```python
from build123d import *

# Parameters (mm, degrees)
BOSS_EXTRUDE1_DEPTH      = 2.5
CHAMFER1_SIZE            = 2.65
CHAMFER1_SIZE_2          = 0.5
FILLET1_R                = 0.254
REVOLVE1_ANGLE           = 180
REVOLVE1_OTHER_WAY_ANGLE = 180
SKETCH3_W                = 0.4
SKETCH3_H                = 0.76
BOSS_EXTRUDE2_DEPTH      = 4.8


with BuildPart() as part:
    # Sketch1 → Boss-Extrude1 (new body)
    with BuildSketch(Plane(origin=(0, 0, 0), x_dir=(1, 0, 0), z_dir=(0, 1, 0))):
        Polygon((-3.825, -2.325), (-2.325, -3.825), (3.825, -3.825), (3.825, 3.825), (-3.825, 3.825), align=None)
    extrude(amount=BOSS_EXTRUDE1_DEPTH)

    # Chamfer1
    # the kernel refuses this chamfer: 2.65, 0.5 mm, written as the material it takes off along each edge
    with BuildSketch(Plane(origin=(3.825, 2.5, 10.710580639), x_dir=(0.007135648431947453, -0.9999745409366458, 0), z_dir=(0, 0, -1)), Plane(origin=(10.710580639, 2.5, -3.825), x_dir=(0, -0.9999745409366458, -0.007135648431947453), z_dir=(-1, 0, 0))) as chamfer1_piece_1:
        Polygon((CHAMFER1_SIZE * 0.999974540937, CHAMFER1_SIZE * 0.00713564843195), (-CHAMFER1_SIZE_2 * 0.00713564843195, CHAMFER1_SIZE_2 * 0.999974540937), (0, 0), align=None)
    extrude(amount=21.421161277, mode=Mode.SUBTRACT)
    with BuildSketch(Plane(origin=(-3.825, 2.5, -10.710580639), x_dir=(-0.007135648431947453, -0.9999745409366458, 0), z_dir=(0, 0, 1)), Plane(origin=(-9.210580639, 2.5, 3.825), x_dir=(0, -0.9999745409366458, 0.007135648431947453), z_dir=(1, 0, 0))) as chamfer1_piece_2:
        Polygon((CHAMFER1_SIZE * 0.999974540937, CHAMFER1_SIZE * 0.00713564843195), (-CHAMFER1_SIZE_2 * 0.00713564843195, CHAMFER1_SIZE_2 * 0.999974540937), (0, 0), align=None)
    extrude(amount=19.921161277, mode=Mode.SUBTRACT)
    with BuildSketch(Plane(origin=(-8.693840762, 2.5, -2.543840762), x_dir=(-0.0050456653943929935, -0.9999745409366458, 0.005045665394392992), z_dir=(0.7071067811865475, 0, 0.7071067811865476))) as chamfer1_piece_3:
        Polygon((CHAMFER1_SIZE * 0.999974540937, CHAMFER1_SIZE * 0.00713564843195), (-CHAMFER1_SIZE_2 * 0.00713564843195, CHAMFER1_SIZE_2 * 0.999974540937), (0, 0), align=None)
    extrude(amount=15.892481621, mode=Mode.SUBTRACT)

    # Fillet1
    fillet1_edges = [part.edges().sort_by_distance(p)[0] for p in [
        (0.603553391, 2.5, 3.325),
        (-2.721446609, 2.5, 2.721446609),
        (-3.325, 2.5, -0.603553391),
        (0, 2.5, -3.325),
        (3.325, 2.5, 0),
        (-3.560849057, 1.25, 2.215585097),
        (-2.215585097, 1.25, 3.560849057),
        (-3.560849057, 1.25, -3.560849057),
        (3.560849057, 1.25, 3.560849057),
        (3.560849057, 1.25, -3.560849057),
    ]]
    fillet(fillet1_edges, radius=FILLET1_R)

    # Sketch2 → Revolve1 (revolve)
    with BuildSketch(Plane(origin=(0, 2.5, 0), x_dir=(1, 0, 0), z_dir=(0, 1, 0))):
        with BuildLine():
            Line((0, -2.45), (0, 2.45))
            ThreePointArc((0, 2.45), (2.45, 0), (0, -2.45))
        make_face()
    revolve(axis=Axis((0, 2.5, 2.45), (0, 0, -1)), revolution_arc=REVOLVE1_ANGLE)

    # Sketch2 → Revolve1 other way (revolve)
    with BuildSketch(Plane(origin=(0, 2.5, 0), x_dir=(1, 0, 0), z_dir=(0, 1, 0))):
        with BuildLine():
            Line((0, -2.45), (0, 2.45))
            ThreePointArc((0, 2.45), (2.45, 0), (0, -2.45))
        make_face()
    revolve(axis=Axis((0, 2.5, 2.45), (0, 0, 1)), revolution_arc=REVOLVE1_OTHER_WAY_ANGLE)

    # Sketch3 → Boss-Extrude2 (add)
    with BuildSketch(Plane.XZ):
        with Locations((-2.707698113, 2.234442884)):
            Rectangle(SKETCH3_W, SKETCH3_H)
        with Locations((-2.707698113, -2.525557116)):
            Rectangle(SKETCH3_W, SKETCH3_H)
        with Locations((2.712301887, -2.525557116)):
            Rectangle(SKETCH3_W, SKETCH3_H)
        with Locations((2.712301887, 2.234442884)):
            Rectangle(SKETCH3_W, SKETCH3_H)
    extrude(amount=BOSS_EXTRUDE2_DEPTH)


solid = part.part
```
Geometry check sheet. Reference: the model listing, model coordinates, mm. Round coordinates to 2 decimals unless told otherwise and drop trailing zeros. Loops run counter-clockwise (first coordinate to the right, second up) from the corner with the lowest first, then second, coordinate; pieces in that order, holes last. Notation, with made-up numbers: (49.5, 85.25) - (106.5, 85.25) arc R27 cw to (106.5, 106.25) - close; hole circle Ø6 at (-2, 27). An arc over 180 degrees is marked (long way). Use a Markdown table: item, result.
Q1. Cross-section at A-A on y = -2.5. Record the cut outline in (x, z), plus the area to 3 significant figures.
Solutions:
| item | result |
|---|---|
| outline | (-2.91, -2.91) - (-2.51, -2.91) - (-2.51, -2.15) - (-2.91, -2.15) - close; (-2.91, 1.85) - (-2.51, 1.85) - (-2.51, 2.61) - (-2.91, 2.61) - close; (2.51, -2.91) - (2.91, -2.91) - (2.91, -2.15) - (2.51, -2.15) - close; (2.51, 1.85) - (2.91, 1.85) - (2.91, 2.61) - (2.51, 2.61) - close |
| area | 1.22 mm2 |
Q2. Cross-section at C-C on z = 1.25. Record the cut outline in (x, y).
Solutions:
| item | result |
|---|---|
| outline | (-3.8, 0) - (3.8, 0) - (3.36, 2.29) arc R0.25 ccw to (3.11, 2.5) - (2.11, 2.5) arc R2.11 ccw to (-2.11, 2.5) - (-3.11, 2.5) arc R0.25 ccw to (-3.36, 2.29) - close |
Q3. Draft check along X on faces 1 (the flat face through (0.05, 1.13, -3.583)), 2 (the cylindrical face through (-2.68, 2.44, 2.7)), 3 (the flat face through (0, 0, 0)). Enter one of: released by +X, released by -X, zero draft, split by the parting line, or undercut.
Solutions:
| item | result |
|---|---|
| face 1 | zero draft |
| face 2 | released by -X |
| face 3 | undercut |
Q4. Go/stop test with flat-tipped pins: P1, Ø0.8, axis at y = -3, z = -2.5, coming from the +X side; P2, Ø4, axis at x = -2.5, y = -2.5, coming from the -Z side; P3, Ø0.8, axis at y = -2, z = 2, coming from the -X side. Record where each tip stops, or that it passes through.
Solutions:
| item | result |
|---|---|
| P1 | stops at x = 2.91 |
| P2 | stops at z = -2.91 |
| P3 | stops at x = -2.91 |
Q5. Cross-section at D-D on y = 3.25. Record the cut outline in (x, z), plus the area to 3 significant figures.
Solutions:
| item | result |
|---|---|
| outline | circle Ø4.66 at (0, 0) |
| area | 17.1 mm2 |
Q6. Cross-section at B-B on x = 1. Record the cut outline in (y, z).
Solutions:
| item | result |
|---|---|
| outline | (0, -3.8) - (2.29, -3.36) arc R0.25 ccw to (2.5, -3.11) - (2.5, -2.24) arc R2.24 ccw to (2.5, 2.24) - (2.5, 3.11) arc R0.25 ccw to (2.29, 3.36) - (0, 3.8) - close |
Q7. Material ranges on line 1 (X direction, y = -2.5, z = 2.25); line 2 (Y direction, x = 2, z = 2); line 3 (X direction, y = 2, z = -3), recorded low to high.
Solutions:
| item | result |
|---|---|
| line 1 | x = -2.91 to -2.51, 2.51 to 2.91 |
| line 2 | y = 0 to 2.5 |
| line 3 | x = -3.42 to 3.42 |
